Drawing for the job (mm, zero at the part's lowest x, y, z). A direction names the side the tool comes from. Give positions to 0.01 mm unless a question says otherwise; leave off trailing zeros. Loops run counter-clockwise (first coordinate to the right, second up) from the corner with the lowest first, then second, coordinate; pieces in that order, holes last. Notation, with made-up numbers: (32, 17.25) - (83, 17.25) arc R21 ccw to (83, 46.25) - close; hole circle Ø2 at (-7, -34.75). An arc over 180 degrees is marked (long way). Return JSON: item names as keys, results as strings. Group by question number.
1) 3-axis set-ups, long thin cutter, end or side, ignore diameter. For the marked faces 5, 6, 7 and 8: which of +Z, -Z, +X, -X, +Y, -Y reach the whole face in a straight line?
2) Slice it at A-A (x = 32.3). List the corners of the cut face in (y, z).
3) Slice it at C-C (y = 1.75). List the corners of the cut face in (x, z), and give its area (3 significant figures).
4) Drop flat-ended pins along their axis: pin 1 (2.5 mm diameter, centred on x = 5.5, y = 7, fed in from +Z); pin 2 (6 mm diameter, centred on x = 22.5, y = 6, fed in from +Z); pin 3 (0.9 mm diameter, centred on x = 2.5, y = 6.5, fed in from -Z); pin 4 (1.4 mm diameter, centred on x = 32.5, y = 6.5, fed in from +Z). Give the stop position or say it passes through.
5) Drill centre lines: probe 1 along Y at (x, z) = (4.7, 19.65); probe 2 along Z at (x, y) = (26.5, 3); probe 3 along Y at (x, z) = (5.5, 20.5). Where is each one in solid material? Low to high. Write a range as from..to.
6) Slice it at D-D (z = 16). List the corners of the cut face in (x, y).
7) Mould opens along Z. For the marked faces 1, 2, 3 and 4 say: released by +Z, released by -Z, zero draft, split by the parting line, or undercut.
8) Slice it at B-B (x = 4.7). List the corners of the cut face in (y, z).
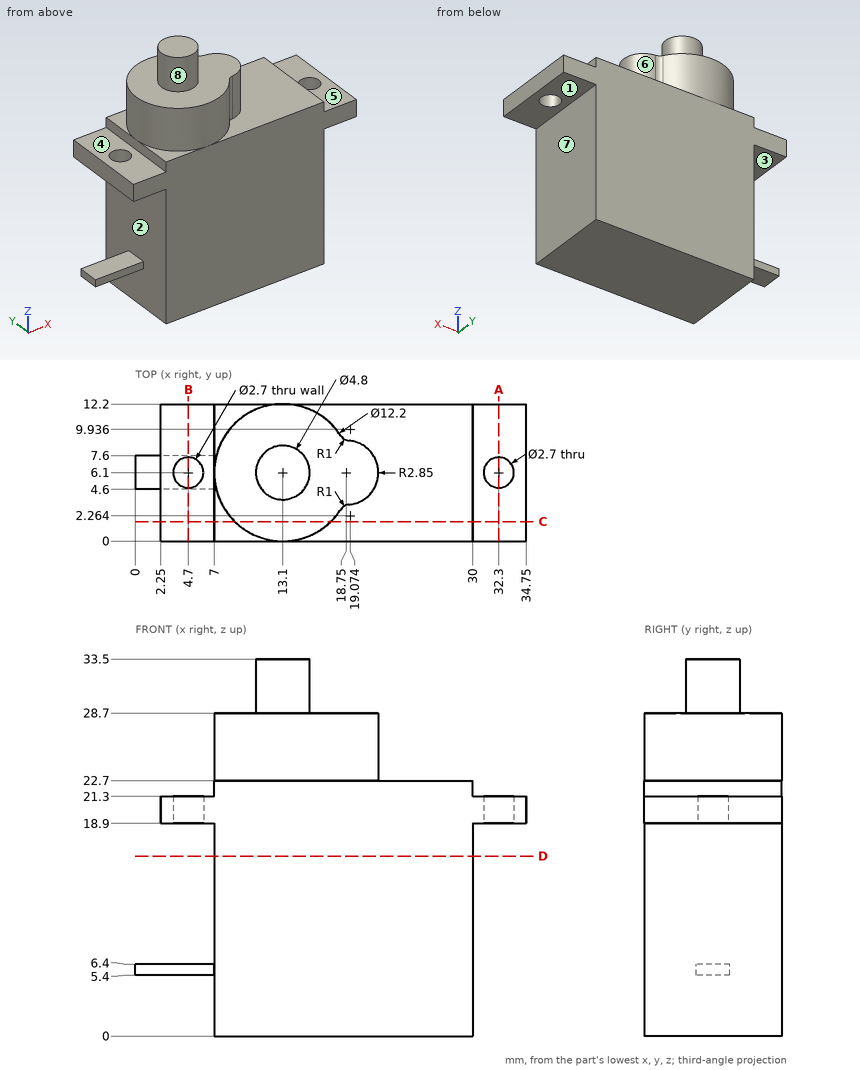
Results:
{
 "1": {"face 5": "+Z, +X, +Y, -Y", "face 6": "+Z, +X", "face 7": "-Z, +X, +Y, -Y", "face 8": "+Z"},
 "2": {"outline": "(0, 18.9) - (4.75, 18.9) - (4.75, 21.3) - (0, 21.3) - close; (7.45, 18.9) - (12.2, 18.9) - (12.2, 21.3) - (7.45, 21.3) - close"},
 "3": {"outline": "(2.25, 18.9) - (7, 18.9) - (7, 0) - (30, 0) - (30, 18.9) - (34.75, 18.9) - (34.75, 21.3) - (30, 21.3) - (30, 22.7) - (17.38, 22.7) - (17.38, 28.7) - (8.82, 28.7) - (8.82, 22.7) - (7, 22.7) - (7, 21.3) - (2.25, 21.3) - close", "area": "596 mm2"},
 "4": {"pin 1": "z = 21.3", "pin 2": "z = 28.7", "pin 3": "z = 5.4", "pin 4": "through"},
 "5": {"probe 1": "0..4.75, 7.45..12.2", "probe 2": "0..22.7", "probe 3": "0..5.01, 7.19..12.2"},
 "6": {"outline": "(7, 0) - (30, 0) - (30, 12.2) - (7, 12.2) - close"},
 "7": {"face 1": "released by -Z", "face 2": "undercut", "face 3": "undercut", "face 4": "released by +Z"},
 "8": {"outline": "(0, 18.9) - (4.75, 18.9) - (4.75, 21.3) - (0, 21.3) - close; (4.6, 5.4) - (7.6, 5.4) - (7.6, 6.4) - (4.6, 6.4) - close; (7.45, 18.9) - (12.2, 18.9) - (12.2, 21.3) - (7.45, 21.3) - close"}
}
